Read the model definition and answer for the solid it produces. Units are mm, in the model's axes. Give positions to 0.01 mm unless a question says otherwise; leave off trailing zeros. Order: outer loops, then holes, each group sorted by start corner. A loop starts at its lowest first (then second) coordinate and runs counter-clockwise, first axis right, second up. Notation, with made-up numbers: (72, 55) -> (109, 55) arc R15 cw to (109, 70) -> close; hole circle Ø7 at (-38.5, -32.5). An arc over 180 degrees is marked (long way). One line per item, written item: value. Start each with the question number.
from build123d import *

# Parameters (mm, degrees)
SKETCH_1_W          = 95
SKETCH_1_H          = 56
SKETCH_1_R          = 1.6
EXTRUDE_1_DEPTH     = 3
FILLET_1_R          = 6
SKETCH_2_W          = 20
SKETCH_2_H          = 3
CUT_EXTRUDE_1_DEPTH = 4
FILLET_2_R          = 2
FILLET_3_R          = 1


with BuildPart() as part:
    # 草图1 → 凸台-拉伸1 (new body)
    with BuildSketch(Plane(origin=(0, 0, 0), x_dir=(1, 0, 0), z_dir=(0, 1, 0))):
        Rectangle(SKETCH_1_W, SKETCH_1_H)
        with Locations((-40.5, 22.5)):
            Circle(SKETCH_1_R, mode=Mode.SUBTRACT)
        with Locations((-40.5, -22.5)):
            Circle(SKETCH_1_R, mode=Mode.SUBTRACT)
        with Locations((40.5, -22.5)):
            Circle(SKETCH_1_R, mode=Mode.SUBTRACT)
        with Locations((40.5, 22.5)):
            Circle(SKETCH_1_R, mode=Mode.SUBTRACT)
    extrude(amount=EXTRUDE_1_DEPTH)

    # 圆角1
    fillet_1_edges = [part.edges().sort_by_distance(p)[0] for p in [
        (47.5, 1.5, 28),
        (-47.5, 1.5, 28),
        (-47.5, 1.5, -28),
        (47.5, 1.5, -28),
    ]]
    fillet(fillet_1_edges, radius=FILLET_1_R)

    # 草图2 → 切除-拉伸1 (cut, through all)
    with BuildSketch(Plane(origin=(0, 3, 0), x_dir=(1, 0, 0), z_dir=(0, 1, 0))):
        with Locations((26, 24)):
            Rectangle(SKETCH_2_W, SKETCH_2_H)
        with Locations((-26, 24)):
            Rectangle(SKETCH_2_W, SKETCH_2_H)
        with Locations((-26, -24)):
            Rectangle(SKETCH_2_W, SKETCH_2_H)
        with Locations((26, -24)):
            Rectangle(SKETCH_2_W, SKETCH_2_H)
        Polygon((-39.458110344, 0), (-24.878897572, 19), (-29.920787228, 19), (-44.5, 0), (-29.920787228, -19), (-24.878897572, -19), align=None)
        Polygon((-19.920787228, -19), (-14.878897572, -19), (-29.458110344, 0), (-14.878897572, 19), (-19.920787228, 19), (-34.5, 0), align=None)
        Polygon((-9.920787228, -19), (-4.878897572, -19), (-19.458110344, 0), (-4.878897572, 19), (-9.920787228, 19), (-24.5, 0), align=None)
        Polygon((44.5, 0), (29.920787228, -19), (24.878897572, -19), (39.458110344, 0), (24.878897572, 19), (29.920787228, 19), align=None)
        Polygon((34.5, 0), (19.920787228, -19), (14.878897572, -19), (29.458110344, 0), (14.878897572, 19), (19.920787228, 19), align=None)
        Polygon((24.5, 0), (9.920787228, -19), (4.878897572, -19), (19.458110344, 0), (4.878897572, 19), (9.920787228, 19), align=None)
        Polygon((-14.579212772, 0), (0, 19), (14.579212772, 0), (0, -18), align=None)
    extrude(amount=-CUT_EXTRUDE_1_DEPTH, mode=Mode.SUBTRACT)

    # 圆角2
    fillet_2_edges = [part.edges().sort_by_distance(p)[0] for p in [
        (0, 1.5, 18),
        (-14.579212772, 1.5, 0),
        (0, 1.5, -19),
        (14.579212772, 1.5, 0),
    ]]
    fillet(fillet_2_edges, radius=FILLET_2_R)

    # 圆角3
    fillet_3_edges = [part.edges().sort_by_distance(p)[0] for p in [
        (36, 1.5, -25.5),
        (36, 1.5, -22.5),
        (16, 1.5, -22.5),
        (16, 1.5, -25.5),
        (-36, 1.5, 25.5),
        (-36, 1.5, 22.5),
        (-16, 1.5, 22.5),
        (-16, 1.5, 25.5),
        (16, 1.5, 22.5),
        (36, 1.5, 22.5),
        (36, 1.5, 25.5),
        (16, 1.5, 25.5),
        (-16, 1.5, -25.5),
        (-16, 1.5, -22.5),
        (-36, 1.5, -22.5),
        (-36, 1.5, -25.5),
    ]]
    fillet(fillet_3_edges, radius=FILLET_3_R)


solid = part.part
Item 1: Find the intervals of material crossed by line 1 (Z direction, x = -40.5, y = 0.7); line 2 (X direction, y = 0.35, z = 21.5); line 3 (Z direction, x = 6.5, y = 1.3), in increasing order. Write a range as from..to.
Item 2: Find section A-A on x = -38. Write down the section's boundary in (y, z), then the cut area to 3 significant figures.
Item 3: Find section C-C on x = 28.5. Write down the section's boundary in (y, z), then the cut area to 3 significant figures.
Item 4: For a pull along Z with two mould halves and no side action, classify faces 1 (the flat face through (-26, 2, 22.5)), 2 (the flat face through (26, 2, 25.5)), 3 (the flat face through (-1, 1, 28)) as +Z half, -Z half, draft (parallel to the pull), parting line (faces both ways), or undercut.
Item 5: Flat-ended cylindrical pins translate along their axes: pin 1 (3 mm diameter, centred on x = -40.5, z = 22.5, fed in from -Y); pin 2 (0.8 mm diameter, centred on y = 2, z = 24, fed in from +X); pin 3 (0.5 mm diameter, centred on y = 1.5, z = -24, fed in from -X). Find the tip coordinate at first contact, or state that the pin passes through.
Item 6: Find section B-B on z = 10.5. Count the separate pieces of the cut face and the enclosed holes in it, then the cut area to 3 significant figures.
Checks:
1. line 1: -28..-24.1, -20.9..-5.21, 5.21..20.9, 24.1..28
1. line 2: -47.5..-41.75, -39.25..39.25, 41.75..47.5
1. line 3: -28..-19, -16.89..-10.53, 9.97..16.89, 19..28
2. outline: (0, -28) -> (3, -28) -> (3, -8.47) -> (0, -8.47) -> close; (0, -1.9) -> (3, -1.9) -> (3, 1.9) -> (0, 1.9) -> close; (0, 8.47) -> (3, 8.47) -> (3, 28) -> (0, 28) -> close
2. area: 129 mm2
3. outline: (0, -28) -> (3, -28) -> (3, -25.5) -> (0, -25.5) -> close; (0, -22.5) -> (3, -22.5) -> (3, -19) -> (0, -19) -> close; (0, -14.28) -> (3, -14.28) -> (3, -7.82) -> (0, -7.82) -> close; (0, -1.25) -> (3, -1.25) -> (3, 1.25) -> (0, 1.25) -> close; (0, 7.82) -> (3, 7.82) -> (3, 14.28) -> (0, 14.28) -> close; (0, 19) -> (3, 19) -> (3, 22.5) -> (0, 22.5) -> close; (0, 25.5) -> (3, 25.5) -> (3, 28) -> (0, 28) -> close
3. area: 82.3 mm2
4. face 1: undercut
4. face 2: undercut
4. face 3: +Z half
5. pin 1: through
5. pin 2: x = 47.28
5. pin 3: x = -47.24
6. separate pieces: 8
6. enclosed holes: 0
6. area: 158 mm2
